```python
from build123d import *
from OCP.BRepFilletAPI import BRepFilletAPI_MakeChamfer

# Parameters (mm, degrees)
SKETCH_1_W                = 150
SKETCH_1_H                = 60
EXTRUDE_1_DEPTH           = 100
SKETCH_5_R                = 2.25
CUT_EXTRUDE_5_DEPTH       = 191
CUT_EXTRUDE_7_DEPTH       = 50
CUT_EXTRUDE_8_DEPTH       = 191
SKETCH_10_R               = 2.25
CUT_EXTRUDE_9_DEPTH       = 191
SKETCH_11_R               = 6
CUT_EXTRUDE_10_DEPTH      = 50
FILLET_1_R                = 10
CHAMFER_2_SIZE            = 10
CHAMFER_2_SIZE_2          = 17.320508076
CHAMFER_4_SIZE            = 5
CHAMFER_4_SIZE2           = 8.660254038
CUT_EXTRUDE_11_DEPTH      = 10
CUT_EXTRUDE_11_DEPTH_BACK = 3
SKETCH_12_R               = 4.5


with BuildPart() as part:
    # 草图1 → 凸台-拉伸1 (new body)
    with BuildSketch(Plane.XY):
        with Locations((75, 30)):
            Rectangle(SKETCH_1_W, SKETCH_1_H)
    extrude(amount=EXTRUDE_1_DEPTH)

    # 草图5 → 切除-拉伸5 (cut, through all)
    with BuildSketch(Plane.XY.offset(100)):
        with Locations((6, 45)):
            Circle(SKETCH_5_R)
        with Locations((6, 15)):
            Circle(SKETCH_5_R)
    extrude(amount=-CUT_EXTRUDE_5_DEPTH, mode=Mode.SUBTRACT)

    # 草图8 → 切除-拉伸7 (cut)
    with BuildSketch(Plane.XZ):
        with BuildLine():
            Line((124.5, 55), (124.5, 100))
            Line((124.5, 100), (19.5, 100))
            Line((19.5, 100), (35.436672603, 40.523528143))
            Line((35.436672603, 40.523528143), (61.556942546, 22.233918228))
            ThreePointArc((61.556942546, 22.233918228), (102.969944529, 19.519566673), (124.5, 55))
        make_face()
    extrude(amount=-CUT_EXTRUDE_7_DEPTH, mode=Mode.SUBTRACT)

    # 草图9 → 切除-拉伸8 (cut, through all)
    with BuildSketch(Plane.XZ):
        with BuildLine():
            Line((150, 80), (150, 0))
            Line((150, 0), (99.466629547, 0))
            ThreePointArc((99.466629547, 0), (124.98259213, 14.873204284), (139.629974877, 40.519465822))
            Line((139.629974877, 40.519465822), (150, 80))
        make_face()
        Polygon((19.621472223, 30), (27.659947996, 0), (0, 0), (0, 30), align=None)
    extrude(amount=-CUT_EXTRUDE_8_DEPTH, mode=Mode.SUBTRACT)

    # 草图10 → 切除-拉伸9 (cut, through all)
    with BuildSketch(Plane(origin=(0, 60, 0), x_dir=(1, 0, 0), z_dir=(0, 1, 0))):
        with Locations(Location((30, -55, 0), (0, 0, 270))):
            Circle(SKETCH_10_R)
        with Locations(Location((60, -85, 0), (0, 0, 270))):
            Circle(SKETCH_10_R)
    extrude(amount=-CUT_EXTRUDE_9_DEPTH, mode=Mode.SUBTRACT)

    # 草图11 → 切除-拉伸10 (cut)
    with BuildSketch(Plane.XZ):
        with Locations((30, 55)):
            Circle(SKETCH_11_R)
    extrude(amount=-CUT_EXTRUDE_10_DEPTH, mode=Mode.SUBTRACT)

    # 圆角1
    fillet_1_edges = [part.edges().sort_by_distance(p)[0] for p in [
        (32.956659097, 25, 49.779064549),
        (29.950074163, 25, 60.999792281),
    ]]
    fillet(fillet_1_edges, radius=FILLET_1_R)

    # 倒角2
    # the kernel refuses this chamfer: 17.320508076, 10 mm, written as the material it adds along each edge
    with BuildSketch(Plane(origin=(-1.269235366, 50, 66.225281599), x_dir=(-0.0332065552835215, -0.9983227437537926, -0.04742387573893358), z_dir=(0.8191520442889948, 0, -0.5735764363510419))) as chamfer_2_piece_1_section:
        Polygon((CHAMFER_2_SIZE * 0.998322743754, -CHAMFER_2_SIZE * 0.0578938624027), (-CHAMFER_2_SIZE_2 * 0.0578938624016, -CHAMFER_2_SIZE_2 * 0.998322743736), (0, 0), align=None)
    chamfer_2_piece_1 = extrude(amount=76.696601504, mode=Mode.PRIVATE)
    chamfer_2_piece_1 = split(chamfer_2_piece_1, bisect_by=Plane(origin=(0, 46.853516386, 53.66836115), z_dir=(1, 0, 0)), keep=Keep.TOP, mode=Mode.PRIVATE)
    chamfer_2_piece_1 = chamfer_2_piece_1 - Plane(origin=(6, 45, 53.66836115), x_dir=(1, 0, 0), z_dir=(0, 0, 1)) * Cylinder(2.25, 223, mode=Mode.PRIVATE)
    chamfer_2_piece_1 = chamfer_2_piece_1 - Plane(origin=(30, 46.853516386, 55), x_dir=(0, 0, 1), z_dir=(0, 1, 0)) * Cylinder(2.25, 223, mode=Mode.PRIVATE)
    add(chamfer_2_piece_1)
    with BuildSketch(Plane(origin=(124.5, 50, 55), x_dir=(0.05789386240267183, -0.9983227437537926, 0), z_dir=(0, 0, 1))) as chamfer_2_piece_2:
        Polygon((CHAMFER_2_SIZE * 0.998322743754, -CHAMFER_2_SIZE * 0.0578938624027), (-CHAMFER_2_SIZE_2 * 0.0578938624016, -CHAMFER_2_SIZE_2 * 0.998322743736), (0, 0), align=None)
    extrude(amount=45)
    with BuildSketch(Plane(origin=(84.5, 50, 55), x_dir=(-0.5735764363510413, 0, -0.8191520442889951), z_dir=(-0.8191520442889951, 0, 0.5735764363510413))) as chamfer_2_piece_3:
        Polygon((40, CHAMFER_2_SIZE), (40 - CHAMFER_2_SIZE_2, 0), (40, 0), align=None)
    revolve(axis=Axis((84.5, 50, 55), (0, -1, 0)), revolution_arc=125)

    # 倒角3
    # the kernel refuses this chamfer: 33.46065215, 17.320508076, 10 mm, written as the material it takes off along each edge
    with BuildSketch(Plane(origin=(27.659947996, -34.755198876, 0), x_dir=(-0.2684337130154822, 0, 0.9632981582649901), z_dir=(0, 1, 0))) as chamfer_3_piece_1_section:
        with BuildLine():
            Line((34.755198876, 0), (-3.980545955, 9.966488807))
            Line((-3.980545955, 9.966488807), (-4.625197647, 9.786849465))
            ThreePointArc((-4.625197647, 9.786849465), (-2.076639928, 4.959177295), (-0.644651692, -0.179639342))
            Line((-0.644651692, -0.179639342), (0.006670144, -0.669179801))
            ThreePointArc((0.006670144, -0.669179801), (17.382543222, -0.495983324), (34.76186902, -0.669179801))
            Line((34.76186902, -0.669179801), (34.755198876, 0))
        make_face()
    chamfer_3_piece_1 = extrude(amount=129.510397752, mode=Mode.PRIVATE)
    chamfer_3_piece_1 = split(chamfer_3_piece_1, bisect_by=Plane(origin=(27.837157989, 30, 30), z_dir=(0, 0, -1)), keep=Keep.TOP, mode=Mode.PRIVATE)
    add(chamfer_3_piece_1, mode=Mode.SUBTRACT)
    with BuildSketch(Plane(origin=(139.629974877, 60, 40.519465822), x_dir=(0.05599451192610632, -0.9983227437537928, -0.014707614968315207), z_dir=(0.2540444592557946, 0, 0.9671925417006848))) as chamfer_3_piece_2:
        with BuildLine():
            Line((10.363792898, 0), (-1.383316572, -17.870395769))
            Line((-1.383316572, -17.870395769), (-1.729145715, -17.850340747))
            ThreePointArc((-1.729145715, -17.850340747), (-0.864572857, -8.925170374), (-0.345829143, 0.020055022))
            Line((-0.345829143, 0.020055022), (0.020055022, 0.345829143))
            ThreePointArc((0.020055022, 0.345829143), (5.184583312, 0.04633232), (10.38384792, 0.345829143))
            Line((10.38384792, 0.345829143), (10.363792898, 0))
        make_face()
    extrude(amount=58.743581506, mode=Mode.SUBTRACT)
    with BuildSketch(Plane(origin=(84.5, 60, 55), x_dir=(-0.0488032324708506, 0, -0.9988084123095861), z_dir=(-0.9988084123095861, 0, 0.0488032324708506))) as chamfer_3_piece_3:
        with BuildLine():
            Line((57.6, 10.346410162), (39.079491924, -0.346410162))
            Line((39.079491924, -0.346410162), (39.079491924, -0.692820323))
            ThreePointArc((39.079491924, -0.692820323), (48.039745962, -0.346410162), (57, -0.346410162))
            Line((57, -0.346410162), (57.346410162, 0))
            ThreePointArc((57.346410162, 0), (57.346410162, 5.173205081), (57.946410162, 10.346410162))
            Line((57.946410162, 10.346410162), (57.6, 10.346410162))
        make_face()
    revolve(axis=Axis((84.5, 60, 55), (0, -1, 0)), revolution_arc=78.080358164, mode=Mode.SUBTRACT)
    with BuildSketch(Plane(origin=(150, 60, 62.076144118), x_dir=(0.057893862402670464, -0.9983227437537926, 0), z_dir=(0, 0, 1))) as chamfer_3_piece_4:
        with BuildLine():
            Line((10.363792898, 0), (-1.383316572, -17.870395769))
            Line((-1.383316572, -17.870395769), (-1.729145715, -17.850340747))
            ThreePointArc((-1.729145715, -17.850340747), (-0.864572857, -8.925170374), (-0.345829143, 0.020055022))
            Line((-0.345829143, 0.020055022), (0.020055022, 0.345829143))
            ThreePointArc((0.020055022, 0.345829143), (5.184583312, 0.04633232), (10.38384792, 0.345829143))
            Line((10.38384792, 0.345829143), (10.363792898, 0))
        make_face()
    extrude(amount=55.847711765, mode=Mode.SUBTRACT)
    # the kernel refuses this chamfer: 33.46065215, 17.320508076, 10 mm, written as the material it takes off along each edge
    with BuildSketch(Plane(origin=(99.736475847, 60, 0), x_dir=(0, -0.9983227437537926, -0.05789386240267141), z_dir=(-1, 0, 0))) as chamfer_3_2_piece_1:
        with BuildLine():
            Line((10.363792898, 0), (-1.383316572, 17.870395769))
            Line((-1.383316572, 17.870395769), (-1.729145715, 17.850340747))
            ThreePointArc((-1.729145715, 17.850340747), (-0.864572857, 8.925170374), (-0.345829143, -0.020055022))
            Line((-0.345829143, -0.020055022), (0.020055022, -0.345829143))
            ThreePointArc((0.020055022, -0.345829143), (5.184583312, -0.04633232), (10.38384792, -0.345829143))
            Line((10.38384792, -0.345829143), (10.363792898, 0))
        make_face()
    extrude(amount=80.000383734, mode=Mode.SUBTRACT)

    # 倒角4: one chamfer whose edges measure the first distance from different faces: ONE call of the kernel's chamfer builder (chamfer() names one face for all edges)
    chamfer_4_edges_1 = [part.edges().sort_by_distance(p)[0] for p in [
        (68.563288771, 0, 0),
    ]]
    chamfer_4_side_1 = [part.faces().sort_by_distance(p)[0] for p in [
        (68.563288771, 25, 0),
    ]]
    chamfer_4_edges_2 = [part.edges().sort_by_distance(p)[0] for p in [
        (124.98259213, 0, 14.873204284),
    ]]
    chamfer_4_side_2 = [part.faces().sort_by_distance(p)[0] for p in [
        (124.98259213, 25, 14.873204284),
    ]]
    chamfer_4_edges_3 = [part.edges().sort_by_distance(p)[0] for p in [
        (144.814987438, 0, 60.259732911),
    ]]
    chamfer_4_side_3 = [part.faces().sort_by_distance(p)[0] for p in [
        (144.814987438, 25, 60.259732911),
    ]]
    chamfer_4_edges_4 = [part.edges().sort_by_distance(p)[0] for p in [
        (150, 0, 90),
    ]]
    chamfer_4_side_4 = [part.faces().sort_by_distance(p)[0] for p in [
        (31.203351809, 0, 45.395528881),
    ]]
    chamfer_4 = BRepFilletAPI_MakeChamfer(part.part.solid().wrapped)
    for e in chamfer_4_edges_1:
        chamfer_4.Add(CHAMFER_4_SIZE, CHAMFER_4_SIZE2, e.wrapped, chamfer_4_side_1[0].wrapped)  # the first distance lies on this face
    for e in chamfer_4_edges_2:
        chamfer_4.Add(CHAMFER_4_SIZE, CHAMFER_4_SIZE2, e.wrapped, chamfer_4_side_2[0].wrapped)  # the first distance lies on this face
    for e in chamfer_4_edges_3:
        chamfer_4.Add(CHAMFER_4_SIZE, CHAMFER_4_SIZE2, e.wrapped, chamfer_4_side_3[0].wrapped)  # the first distance lies on this face
    for e in chamfer_4_edges_4:
        chamfer_4.Add(CHAMFER_4_SIZE, CHAMFER_4_SIZE2, e.wrapped, chamfer_4_side_4[0].wrapped)  # the first distance lies on this face
    add(Compound.cast(chamfer_4.Shape()), mode=Mode.REPLACE)

    # 草图12 → 切除-拉伸11 (cut, two sides: drawn at the far end of the back side and taken through both)
    with BuildSketch(Plane.XZ.offset(-50).offset(-CUT_EXTRUDE_11_DEPTH_BACK)):
        with Locations(Location((30, 55, 0), (0, 0, 55))):
            Circle(SKETCH_12_R)
        with Locations(Location((60, 85, 0), (0, 0, 270))):
            Circle(SKETCH_12_R)
    extrude(amount=CUT_EXTRUDE_11_DEPTH + CUT_EXTRUDE_11_DEPTH_BACK, mode=Mode.SUBTRACT)


solid = part.part
```
Verification items for the finished model (mm, model axes). A direction names the side the tool comes from. Give positions to 0.01 mm unless a question says otherwise; leave off trailing zeros. Loops run counter-clockwise (first coordinate to the right, second up) from the corner with the lowest first, then second, coordinate; pieces in that order, holes last. Notation, with made-up numbers: M -16,27 L 36,27 A38 cw 36,65 Z; hole C -1.75,72.25 d5. An arc over 180 degrees is marked long. One line per question, with ' | ' between items.
Item 1: Thickness scan on line 1 (Y direction, x = 6, z = 84); line 2 (X direction, y = 15.5, z = 89); line 3 (X direction, y = 10, z = 66.5). Record the ranges inside material, lowest first. Write a range as [from, to].
Completed:
line 1: y = [0, 12.75], [17.25, 42.75], [47.25, 60] | line 2: x = [0, 3.81], [8.19, 22.45], [124.5, 150] | line 3: x = [0, 28.27], [124.5, 146.45]
Item 2: Depth check by flat-ended pin: P1, Ø1.5, axis at x = 116, y = 9.5, coming from the +Z side; P2, Ø14.5, axis at x = 60, z = 85, coming from the -Y side; P3, Ø1.5, axis at y = 25.5, z = 19, coming from the +X side. Enter the tip coordinate at first touch or a pass-through.
Completed:
P1: stops at z = 31.34 | P2: stops at y = 50 | P3: stops at x = 129.29
Item 3: Section check B-B, the plane x = 30. Record the cut outline in (y, z), plus the area to 3 significant figures.
Completed:
outline: M 0,13.27 L 57.66,13.27 L 60,17.32 L 60,52.75 L 53,52.75 L 53,50.5 L 42.92,50.5 L 41.99,48.53 L 0,48.53 Z; M 47.17,59.5 L 53,59.5 L 53,57.25 L 60,57.25 L 60,100 L 50,100 L 50,65.47 Z | area: 2,590 mm^2
Item 4: Draft check along Z on faces 3 (the face through (117.14, 56.18, 22.17)), 4 (the face through (141.46, 54.93, 89.86)), 5 (the face through (28.006, 24.65, 63.553)). Enter one of: +Z half, -Z half, draft (parallel to the pull), parting line (faces both ways), or undercut.
Completed:
face 3: -Z half | face 4: draft | face 5: undercut
Item 5: Section check A-A, the plane y = 15. Record the cut outline in (x, z).
Completed:
outline: M 0,30 L 3.75,30 L 3.75,100 L 0,100 Z; M 8.25,30 L 20.34,30 L 37.66,0 L 99.47,0 A57 ccw 139.63,40.52 L 150,80 L 150,100 L 124.5,100 L 124.5,55 A40 cw 61.56,22.23 L 35.44,40.52 L 34.96,42.29 A10 ccw 28.24,49.26 A6 cw 25.61,59.09 A10 ccw 27.94,68.49 L 19.5,100 L 8.25,100 Z
Item 6: Section check C-C, the plane z = 85. Record the cut outline in (x, y).
Completed:
outline: M 0,0 L 23.52,0 L 23.52,50 L 55.5,50 L 55.5,53 L 57.75,53 L 57.75,60 L 0,60 Z; M 62.25,53 L 64.5,53 L 64.5,50 L 107.18,50 L 124.5,40 L 124.5,0 L 142.36,0 L 146.26,2.18 L 150,8.66 L 150,50 L 132.68,60 L 62.25,60 Z; hole C 6,15 d4.5; hole C 6,45 d4.5
Item 7: Tool access check on faces 1 (the face through (65.596, 2.465, 4.391)), 2 (the face through (72, 50, 74)). Record the directions out of +Z, -Z, +X, -X, +Y, -Y that give a thin tool (end or side, any length) a straight path to the whole face; none if there is none.
Completed:
face 1: -Z, +X, -X, -Y | face 2: +Z, -Y
Item 8: Section check D-D, the plane z = 63.5. Record the cut outline in (x, y).
Completed:
outline: M 0,0 L 27.99,0 L 27.99,48.4 L 32.82,50 L 107.18,50 L 124.5,40 L 124.5,0 L 136.71,0 L 145.67,5 L 145.67,50 L 127.76,60 L 0,60 Z; hole C 6,15 d4.5; hole C 6,45 d4.5
